Could you check a few things on this model? Use its own coordinates, in mm. Face numbers are marked on the shaded views. A direction names the side the tool comes from. Round coordinates to 2 decimals unless told otherwise and drop trailing zeros. Loops run counter-clockwise (first coordinate to the right, second up) from the corner with the lowest first, then second, coordinate; pieces in that order, holes last.
from build123d import *

# Parameters (mm, degrees)
SKETCH_1_W          = 14
SKETCH_1_H          = 2.6
EXTRUDE_1_DEPTH     = 24.22
CUT_EXTRUDE_START   = -5.36
CUT_EXTRUDE_1_DEPTH = 5.36
CUT_EXTRUDE_2_DEPTH = 5.36
CUT_EXTRUDE_3_DEPTH = 51.214587522
SKETCH_6_R          = 4.815
EXTRUDE_3_DEPTH     = 6
EXTRUDE_4_DEPTH     = 13
SKETCH_10_W         = 11.9
SKETCH_10_H         = 22.9
EXTRUDE_5_DEPTH     = 6.9
CUT_EXTRUDE_START_2 = -18.08
CUT_EXTRUDE_4_DEPTH = 18.08
SKETCH_12_R         = 1.315
CUT_EXTRUDE_5_DEPTH = 50.492132708
SKETCH_13_R         = 1.4
CUT_EXTRUDE_6_DEPTH = 55.836301845
SKETCH_14_R         = 1.45
CUT_EXTRUDE_7_DEPTH = 15.9
EXTRUDE_6_DEPTH     = 13


# Read off the part's stored shape, not the designer's step: 切除-拉伸4
with BuildPart() as part:
    # 草图1 → 凸台-拉伸1 (new body)
    with BuildSketch(Plane(origin=(0, 0, 0), x_dir=(0, 0, -1), z_dir=(1, 0, 0))):
        with Locations((2.04, 38.8)):
            Rectangle(SKETCH_1_W, SKETCH_1_H)
        Polygon((-9.04, 33.15), (-9.04, -3.4), (9.04, -3.4), (9.04, 37.5), (-4.96, 37.5), (-4.96, 33.15), align=None)
        Polygon((-4.96, 33.15), (-9.04, 33.15), (-4.96, 37.5), align=None)
        Polygon((9.04, -3.4), (-9.04, -3.4), (-4.39, -16.885), (9.04, -16.885), align=None)
        with BuildLine():
            Line((9.04, -16.885), (-4.39, -16.885))
            Line((-4.39, -16.885), (-4.39, -33.385))
            ThreePointArc((-4.39, -33.385), (2.325, -26.67), (9.04, -33.385))
            Line((9.04, -33.385), (9.04, -16.885))
        make_face()
        with BuildLine():
            ThreePointArc((9.04, -33.385), (2.325, -26.67), (-4.39, -33.385))
            Line((-4.39, -33.385), (9.04, -33.385))
        make_face()
        with BuildLine():
            Line((9.04, -33.385), (-4.39, -33.385))
            ThreePointArc((-4.39, -33.385), (-2.423222036, -38.133222036), (2.325, -40.1))
            ThreePointArc((2.325, -40.1), (7.073222036, -38.133222036), (9.04, -33.385))
        make_face()
        with BuildLine():
            ThreePointArc((9.04, -33.385), (2.325, -26.67), (-4.39, -33.385))
            Line((-4.39, -33.385), (9.04, -33.385))
        make_face()
        with BuildLine():
            Line((9.04, -33.385), (-4.39, -33.385))
            ThreePointArc((-4.39, -33.385), (-2.423222036, -38.133222036), (2.325, -40.1))
            ThreePointArc((2.325, -40.1), (7.073222036, -38.133222036), (9.04, -33.385))
        make_face()
    extrude(amount=EXTRUDE_1_DEPTH)

    # 草图2 → 切除-拉伸1 (cut)
    with BuildSketch(Plane(origin=(24.22, 0, 0), x_dir=(0, 0, -1), z_dir=(1, 0, 0)).offset(CUT_EXTRUDE_START)):
        with BuildLine():
            Line((9.04, -33.385), (9.04, -16.885))
            Line((9.04, -16.885), (-4.39, -16.885))
            Line((-4.39, -16.885), (-4.39, -33.385))
            ThreePointArc((-4.39, -33.385), (2.325, -40.1), (9.04, -33.385))
        make_face()
    extrude(amount=CUT_EXTRUDE_1_DEPTH, mode=Mode.SUBTRACT)

    # 草图3 → 切除-拉伸2 (cut)
    with BuildSketch(Plane.ZY):
        with BuildLine():
            Line((4.39, -16.885), (-9.04, -16.885))
            Line((-9.04, -16.885), (-9.04, -33.385))
            ThreePointArc((-9.04, -33.385), (-2.325, -40.1), (4.39, -33.385))
            Line((4.39, -33.385), (4.39, -16.885))
        make_face()
    extrude(amount=-CUT_EXTRUDE_2_DEPTH, mode=Mode.SUBTRACT)

    # 草图4 → 切除-拉伸3 (cut, through all)
    with BuildSketch(Plane(origin=(0, 0, -9.04), x_dir=(-1, 0, 0), z_dir=(0, 0, -1))):
        Polygon((-18.86, -16.885), (-24.22, -3.4), (-24.22, -16.885), align=None)
        Polygon((0, -16.885), (0, -3.4), (-5.36, -16.885), align=None)
    extrude(amount=-CUT_EXTRUDE_3_DEPTH, mode=Mode.SUBTRACT)

    # 草图6 → 凸台-拉伸3 (add)
    with BuildSketch(Plane(origin=(24.22, 0, 0), x_dir=(0, 0, -1), z_dir=(1, 0, 0))):
        with Locations((2.305, 26.655)):
            Circle(SKETCH_6_R)
    extrude(amount=EXTRUDE_3_DEPTH)

    # 草图8 → 凸台-拉伸4 (add)
    with BuildSketch(Plane(origin=(0, 0, -9.04), x_dir=(-1, 0, 0), z_dir=(0, 0, -1))):
        with BuildLine():
            Line((-11.3, 0.85), (-11.3, 18.1))
            Line((-11.3, 18.1), (-11.3, 35.35))
            ThreePointArc((-11.3, 35.35), (-18.385253719, 33.827736002), (-24.22, 29.529615042))
            Line((-24.22, 29.529615042), (-24.22, 6.670384958))
            ThreePointArc((-24.22, 6.670384958), (-18.385253719, 2.372263998), (-11.3, 0.85))
        make_face()
        with BuildLine():
            Line((-24.22, 6.670384958), (-24.22, 29.529615042))
            ThreePointArc((-24.22, 29.529615042), (-28.55, 18.1), (-24.22, 6.670384958))
        make_face()
    extrude(amount=EXTRUDE_4_DEPTH)

    # 草图10 → 凸台-拉伸5 (add)
    with BuildSketch(Plane.XY.offset(9.04)):
        with Locations((11.81, 12.75)):
            Rectangle(SKETCH_10_W, SKETCH_10_H)
    extrude(amount=EXTRUDE_5_DEPTH)

    # 切除-拉伸4 outline → 切除-拉伸4 (cut)
    with BuildSketch(Plane(origin=(0, 0, -9.04), x_dir=(-1, 0, 0), z_dir=(0, 0, -1)).offset(CUT_EXTRUDE_START_2)):
        with BuildLine():
            Line((-9.3, 24.2), (-5.86, 24.2))
            Line((-5.86, 24.2), (-5.86, 1.3))
            Line((-5.86, 1.3), (-9.3, 1.3))
            Line((-9.3, 1.3), (-9.3, -1.045821999))
            ThreePointArc((-9.3, -1.045821999), (-16.054192627, -0.553690049), (-22.22, 2.247047594))
            Line((-22.22, 2.247047594), (-22.22, -3.017090844))
            Line((-22.22, -3.017090844), (-16.86, -16.502090844))
            Line((-16.86, -16.502090844), (-16.86, -39.946221742))
            Line((-16.86, -39.946221742), (-7.36, -39.946221742))
            Line((-7.36, -39.946221742), (-7.36, -16.502090844))
            Line((-7.36, -16.502090844), (-2, -3.017090844))
            Line((-2, -3.017090844), (-2, 38.1))
            Line((-2, 38.1), (-9.3, 38.1))
            Line((-9.3, 38.1), (-9.3, 24.2))
        make_face()
    extrude(amount=CUT_EXTRUDE_4_DEPTH, mode=Mode.SUBTRACT)

    # 草图12 → 切除-拉伸5 (cut, through all)
    with BuildSketch(Plane(origin=(18.86, 0, 0), x_dir=(0, 0, -1), z_dir=(1, 0, 0))):
        with Locations((2.325, -33.385)):
            Circle(SKETCH_12_R)
    extrude(amount=-CUT_EXTRUDE_5_DEPTH, mode=Mode.SUBTRACT)

    # 草图13 → 切除-拉伸6 (cut, through all)
    with BuildSketch(Plane.ZY):
        with Locations(Location((-1, 2.46, 0), (0, 0, 304.04773237))):
            Circle(SKETCH_13_R)
    extrude(amount=-CUT_EXTRUDE_6_DEPTH, mode=Mode.SUBTRACT)

    # 草图14 → 切除-拉伸7 (cut)
    with BuildSketch(Plane(origin=(0, 40.1, 0), x_dir=(1, 0, 0), z_dir=(0, 1, 0))):
        with Locations(Location((12.11, -1.2, 0), (0, 0, 270))):
            Circle(SKETCH_14_R)
    extrude(amount=-CUT_EXTRUDE_7_DEPTH, mode=Mode.SUBTRACT)

    # 草图15 → 凸台-拉伸6 (add)
    with BuildSketch(Plane(origin=(0, 0, -22.04), x_dir=(-1, 0, 0), z_dir=(0, 0, -1))):
        with BuildLine():
            ThreePointArc((-11.3, 21.71), (-14.91, 18.1), (-11.3, 14.49))
            Line((-11.3, 14.49), (-11.3, 21.71))
        make_face()
        with BuildLine():
            Line((-11.3, 21.71), (-11.3, 14.49))
            ThreePointArc((-11.3, 14.49), (-8.74734452, 15.54734452), (-7.69, 18.1))
            ThreePointArc((-7.69, 18.1), (-8.74734452, 20.65265548), (-11.3, 21.71))
        make_face()
    extrude(amount=-EXTRUDE_6_DEPTH)


solid = part.part
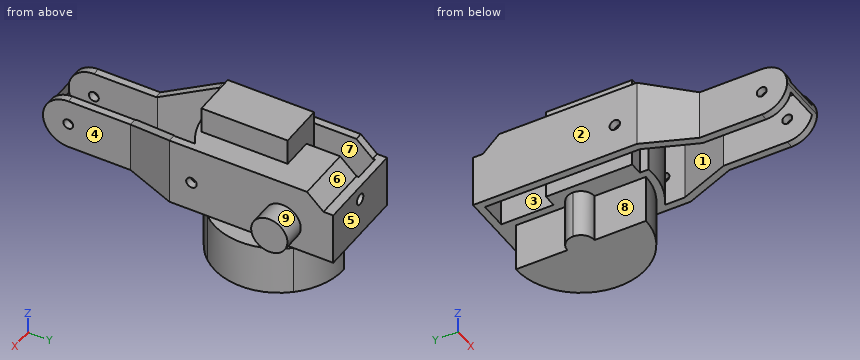
Item 1: We'd pull the mould along X, two halves only. Please class the marked faces 1, 2, 3 and 4: released by +X, released by -X, zero draft, split by the parting line, or undercut.
Results list:
face 1: undercut
face 2: released by -X
face 3: undercut
face 4: released by +X
Item 2: If we section it at A-A, the plane z = -12: Please give me the cut outline in (x, y), then the cut area to 3 significant figures.
Results list:
outline: (11.3, 0.85) arc R17.25 ccw to (11.3, 35.35) - (11.3, 21.71) arc R3.61 ccw to (11.3, 14.49) - close
area: 488 mm2
Item 3: If we section it at B-B, the plane x = 12.11: Please give me the cut outline in (y, z) (3 decimals).
Results list:
outline: (-39.946, -3.754) - (-39.946, -0.896) arc R6.715 ccw to start; (-1.133, -9.04) - (0.869, -9.04) - (0.869, -22.04) - (35.331, -22.04) - (35.331, -9.04) - (40.1, -9.04) - (40.1, -0.25) - (24.2, -0.25) - (24.2, 2.65) - (40.1, 2.65) - (40.1, 4.96) - (37.5, 4.96) - (33.15, 9.04) - (24.2, 9.04) - (24.2, 15.94) - (1.3, 15.94) - (1.3, 9.04) - (-1.133, 9.04) - close; hole circle Ø2.8 at (2.46, -1)
Item 4: If we section it at D-D, the plane z = 6: Please give me the cut outline in (x, y).
Results list:
outline: (0, -3.4) - (3.5, -12.22) - (5.66, -12.22) - (2, -3.02) - (2, 36.39) - (0, 36.39) - close; (5.86, 1.3) - (9.3, 1.3) - (9.3, -1.05) arc R19.25 ccw to (22.22, 2.25) - (22.22, -3.02) - (18.56, -12.22) - (20.72, -12.22) - (24.22, -3.4) - (24.22, 36.39) - (9.3, 36.39) - (9.3, 24.2) - (5.86, 24.2) - close
Item 5: Will these pins go through, and if not, where does the flat tip stop? pin 1 (2.5 mm diameter, centred on x = 12.11, z = 1.2, fed in from +Y); pin 2 (3 mm diameter, centred on x = 7.5, z = -5.5, fed in from -Y); pin 3 (1.7 mm diameter, centred on y = 2.46, z = -1, fed in from -X); pin 4 (1.5 mm diameter, centred on x = 15.5, z = -4, fed in from -Y).
Results list:
pin 1: stops at y = 24.2
pin 2: stops at y = -39.89
pin 3: passes through
pin 4: stops at y = -40.04
Item 6: If I drill on line 1 along X through (y, z) = (32, 1.2); line 2 along X through (y, z) = (24, -4.5); line 3 along Y through (x, z) = (8, -5), over which ranges is the centre line in solid material (lowest first)?
Results list:
line 1: x = 0 to 2, 9.3 to 10.66, 13.56 to 24.22
line 2: x = 0 to 2, 5.86 to 30.22
line 3: y = 1.3 to 24.2, 38.1 to 40.1
Item 7: For the marked faces 5, 6, 7, 8 and 9, which set-ups out of +Z, -Z, +X, -X, +Y, -Y let a thin tool reach every point of the face, with its end or its side?
Results list:
face 5: +Z, -Z, +X, -X, +Y
face 6: +Z, +X, -X, +Y
face 7: +Z, -Z
face 8: -Z, -X, -Y
face 9: +X
Item 8: If we section it at C-C, the plane y = 19: Please give me the cut outline in (x, z), then the cut area to 3 significant figures.
Results list:
outline: (0, -9.04) - (2, -9.04) - (2, 9.04) - (0, 9.04) - close; (5.86, -9.04) - (7.8, -9.04) - (7.8, -22.04) - (28.53, -22.04) - (28.53, -9.04) - (24.22, -9.04) - (24.22, 9.04) - (17.76, 9.04) - (17.76, 15.94) - (5.86, 15.94) - close
area: 720 mm2
